```python
from build123d import *

# Parameters (mm, degrees)
EXTRUDE_1_DEPTH     = 30
SKETCH_2_R          = 10.5
CUT_EXTRUDE_1_DEPTH = 104.903801663
EXTRUDE_3_DEPTH     = 86
SKETCH_5_R          = 4
CUT_EXTRUDE_3_DEPTH = 86
SKETCH_6_R          = 11
CUT_EXTRUDE_4_DEPTH = 5
CUT_EXTRUDE_START   = -5
SKETCH_7_R          = 11
CUT_EXTRUDE_5_DEPTH = 5


with BuildPart() as part:
    # Эскиз1 → Бобышка-Вытянуть1 (new body)
    with BuildSketch(Plane.XY):
        with BuildLine():
            Line((-43, 0), (-43, 30))
            Line((-43, 30), (-35, 30))
            Line((-35, 30), (-35, 50))
            Line((-35, 50), (-25.75, 50))
            Line((-25.75, 50), (-25.75, 42))
            ThreePointArc((-25.75, 42), (-25, 30.04705955), (-24.25, 42))
            Line((-24.25, 42), (-24.25, 50))
            Line((-24.25, 50), (-15, 50))
            Line((-15, 50), (-15, 30))
            Line((-15, 30), (0, 30))
            Line((0, 30), (15, 30))
            Line((15, 30), (15, 50))
            Line((15, 50), (24.25, 50))
            Line((24.25, 50), (24.25, 42))
            ThreePointArc((24.25, 42), (25, 30.04705955), (25.75, 42))
            Line((25.75, 42), (25.75, 50))
            Line((25.75, 50), (35, 50))
            Line((35, 50), (35, 30))
            Line((35, 30), (43, 30))
            Line((43, 30), (43, 0))
            Line((43, 0), (0, 0))
            Line((0, 0), (-43, 0))
        make_face()
    extrude(amount=EXTRUDE_1_DEPTH)

    # Эскиз2 → Вырез-Вытянуть1 (cut, through all)
    with BuildSketch(Plane.ZY.offset(43)):
        with Locations((15.445285693, 13.511926699)):
            Circle(SKETCH_2_R)
    extrude(amount=-CUT_EXTRUDE_1_DEPTH, mode=Mode.SUBTRACT)

    # Эскиз4 → Бобышка-Вытянуть3 (add)
    with BuildSketch(Plane(origin=(43, 0, 0), x_dir=(0, 0, -1), z_dir=(1, 0, 0))):
        Polygon((0, 0), (31.600345964, 0), (31.600345964, 29.791908919), (0, 30), align=None)
    extrude(amount=-EXTRUDE_3_DEPTH)

    # Эскиз5 → Вырез-Вытянуть3 (cut)
    with BuildSketch(Plane.ZY.offset(43)):
        with Locations((-2.905780264, 13.079264153)):
            Circle(SKETCH_5_R)
    extrude(amount=-CUT_EXTRUDE_3_DEPTH, mode=Mode.SUBTRACT)

    # Эскиз6 → Вырез-Вытянуть4 (cut)
    with BuildSketch(Plane.ZY.offset(43)):
        with Locations((-2.905780264, 13.079264153)):
            Circle(SKETCH_6_R)
    extrude(amount=-CUT_EXTRUDE_4_DEPTH, mode=Mode.SUBTRACT)

    # Эскиз7 → Вырез-Вытянуть5 (cut)
    with BuildSketch(Plane(origin=(43, 0, 0), x_dir=(0, 0, -1), z_dir=(1, 0, 0)).offset(CUT_EXTRUDE_START)):
        with Locations((2.905780264, 13.079264153)):
            Circle(SKETCH_7_R)
    extrude(amount=CUT_EXTRUDE_5_DEPTH, mode=Mode.SUBTRACT)


solid = part.part
```
Verification items for the finished model (mm, model axes). A direction names the side the tool comes from. Coordinates: 2 decimals unless noted, no trailing zeros. Loops run counter-clockwise (first coordinate to the right, second up) from the corner with the lowest first, then second, coordinate; pieces in that order, holes last. Notation, with made-up numbers: (82, -35) - (97, -35) arc R23 cw to (97, -9) - close; hole circle Ø10 at (5.25, 21). An arc over 180 degrees is marked (long way). Answer as a JSON object with one key per item and string values.
(1) Mould release check, pull along Y, two halves, no side actions. Record for faces 1 (the cylindrical face through (24.747, 30.052, 14.79)), 2 (the flat face through (20, 50, 15)), 3 (the flat face through (24.25, 46, 15)): pulls with the +Y half, pulls with the -Y half, needs draft (parallel to the pull), parting line crosses it, or undercut.
Response:
{"face 1": "undercut", "face 2": "pulls with the +Y half", "face 3": "needs draft"}
(2) Scan lines: line 1 along X through (y, z) = (47.5, 14.5); line 2 along Z through (x, y) = (24.5, 15); line 3 along Z through (x, y) = (-22, 14). Record each from-to range of solid material in increasing order.
Response:
{"line 1": "x = -35 to -25.75, -24.25 to -15, 15 to 24.25, 25.75 to 35", "line 2": "z = -31.6 to -6.41, 0.6 to 5.05, 25.84 to 30", "line 3": "z = -31.6 to -6.8, 0.99 to 4.96, 25.93 to 30"}
(3) Cross-section at C-C, the plane z = -5. Record the boundary of the cut face in (x, y), then the cut area to 3 significant figures.
Response:
{"outline": "(-43, 0) - (43, 0) - (43, 2.28) - (38, 2.28) - (38, 9.67) - (-38, 9.67) - (-38, 2.28) - (-43, 2.28) - close; (-43, 23.88) - (-38, 23.88) - (-38, 16.49) - (38, 16.49) - (38, 23.88) - (43, 23.88) - (43, 29.97) - (-43, 29.97) - close", "area": "1,840 mm²"}
(4) Cross-section at A-A, the plane y = 5. Record the boundary of the cut face in (x, z), then the cut area to 3 significant figures.
Response:
{"outline": "(-43, -31.6) - (43, -31.6) - (43, -10.37) - (38, -10.37) - (38, 4.56) - (43, 4.56) - (43, 9.3) - (-43, 9.3) - (-43, 4.56) - (-38, 4.56) - (-38, -10.37) - (-43, -10.37) - close; (-43, 21.59) - (43, 21.59) - (43, 30) - (-43, 30) - close", "area": "4,090 mm²"}
(5) Cross-section at B-B, the plane x = -33. Record the boundary of the cut face in (y, z).
Response:
{"outline": "(0, -31.6) - (29.79, -31.6) - (30, 0) - (50, 0) - (50, 30) - (0, 30) - close; hole circle Ø21 at (13.51, 15.45); hole circle Ø8 at (13.08, -2.91)"}
(6) Go/stop test with flat-tipped pins: pin 1 Ø7 at (x, y) = (-25, 36.05) entering from +Z; pin 2 Ø9 at (y, z) = (47.5, 9.5) entering from +X; pin 3 Ø6 at (y, z) = (14, -5) entering from +X; pin 4 Ø9 at (x, z) = (-6.5, 17.5) entering from +Y. Record where each tip stops, or that it passes through.
Response:
{"pin 1": "passes through", "pin 2": "stops at x = 35", "pin 3": "stops at x = 38", "pin 4": "stops at y = 30"}
(7) Cross-section at D-D, the plane x = 36. Record the boundary of the cut face in (y, z), then the cut area to 3 significant figures.
Response:
{"outline": "(0, -31.6) - (29.79, -31.6) - (30, 0) - (30, 30) - (0, 30) - close; hole circle Ø21 at (13.51, 15.45); hole circle Ø8 at (13.08, -2.91)", "area": "1,450 mm²"}
(8) Access from +Z, -Z, +X, -X, +Y, -Y to the whole of each face (thin tool, end or side, straight path). Record for faces 4 (the cylindrical face through (-40.535, 13.222, -13.905)), 5 (the flat face through (-25.75, 46, 15)), 6 (the flat face through (-23, 42, 0)), 7 (the flat face through (-35, 40, 15)), 8 (the flat face through (35, 40, 15)).
Response:
{"face 4": "-X", "face 5": "+Z, -Z, +Y", "face 6": "-Z, +X, -X, +Y", "face 7": "+Z, -Z, -X, +Y", "face 8": "+Z, -Z, +X, +Y"}
